Work out the finished part from the listing and answer in its coordinate system (mm). Face numbers are marked on the shaded views. Give positions to 0.01 mm unless a question says otherwise; leave off trailing zeros. Loops run counter-clockwise (first coordinate to the right, second up) from the corner with the lowest first, then second, coordinate; pieces in that order, holes last.
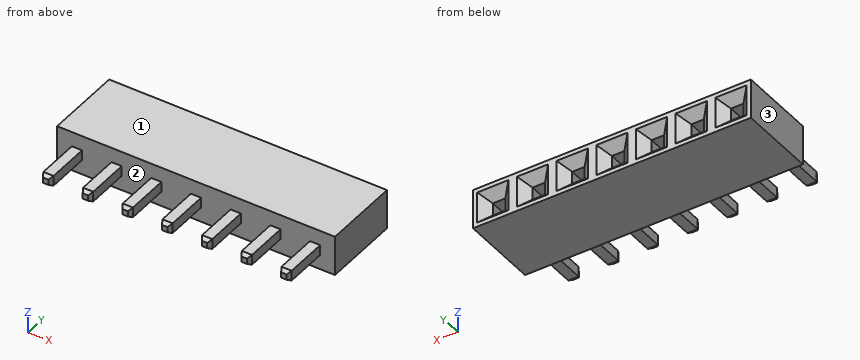
from build123d import *

# Parameters (mm, degrees)
SKETCH1_W                   = 2.54
SKETCH1_H                   = 2.54
BOSS_EXTRUDE1_DEPTH         = 5
SKETCH2_W                   = 0.65
SKETCH2_H                   = 0.65
BOSS_EXTRUDE2_DEPTH         = 3
CHAMFER1_SIZE               = 0.15
CHAMFER1_SIZE2              = 0.259807621
SKETCH3_W                   = 0.8
SKETCH3_H                   = 0.8
CUT_EXTRUDE1_DEPTH          = 3
CHAMFER2_SIZE               = 0.6
LPATTERN1_COUNT             = 7
LPATTERN1_PITCH             = 2.54
CHAMFER1_OF_LPATTERN1_SIZE2 = 0.15
CHAMFER1_OF_LPATTERN1_SIZE  = 0.259807621
CHAMFER2_OF_LPATTERN1_SIZE  = 0.6


with BuildPart() as part:
    # Sketch1 → Boss-Extrude1 (new body)
    with BuildSketch(Plane(origin=(0, 0, 0), x_dir=(1, 0, 0), z_dir=(0, 1, 0))):
        Rectangle(SKETCH1_W, SKETCH1_H)
    boss_extrude1 = extrude(amount=BOSS_EXTRUDE1_DEPTH)

    # Sketch2 → Boss-Extrude2 (add)
    with BuildSketch(Plane.XZ):
        Rectangle(SKETCH2_W, SKETCH2_H)
    boss_extrude2 = extrude(amount=BOSS_EXTRUDE2_DEPTH)

    # Chamfer1
    chamfer1_edges = [part.edges().sort_by_distance(p)[0] for p in [
        (0.325, -3, 0),
        (0, -3, 0.325),
        (-0.325, -3, 0),
        (0, -3, -0.325),
    ]]
    chamfer1_side = [part.faces().sort_by_distance(p)[0] for p in [
        (0, -3, 0),
    ]]
    chamfer(chamfer1_edges, length=CHAMFER1_SIZE, length2=CHAMFER1_SIZE2, reference=chamfer1_side[0])

    # Sketch3 → Cut-Extrude1 (cut)
    with BuildSketch(Plane(origin=(0, 5, 0), x_dir=(1, 0, 0), z_dir=(0, 1, 0))):
        Rectangle(SKETCH3_W, SKETCH3_H)
    cut_extrude1 = extrude(amount=-CUT_EXTRUDE1_DEPTH, mode=Mode.SUBTRACT)

    # Chamfer2
    chamfer2_edges = [part.edges().sort_by_distance(p)[0] for p in [
        (0.4, 5, 0),
        (0, 5, -0.4),
        (-0.4, 5, 0),
        (0, 5, 0.4),
    ]]
    chamfer(chamfer2_edges, length=CHAMFER2_SIZE)

    # LPattern1: Boss-Extrude1, Boss-Extrude2, Cut-Extrude1 ×7
    with Locations(*[(i * LPATTERN1_PITCH, 0, 0) for i in range(1, LPATTERN1_COUNT)]):
        add(boss_extrude1)
        add(boss_extrude2)
        add(cut_extrude1, mode=Mode.SUBTRACT)

    # Chamfer1 of LPattern1
    chamfer1_of_lpattern1_edges = [part.edges().sort_by_distance(p)[0] for p in [
        (2.865, -3, 0),
        (2.54, -3, 0.325),
        (2.215, -3, 0),
        (2.54, -3, -0.325),
        (5.405, -3, 0),
        (5.08, -3, 0.325),
        (4.755, -3, 0),
        (5.08, -3, -0.325),
        (7.945, -3, 0),
        (7.62, -3, 0.325),
        (7.295, -3, 0),
        (7.62, -3, -0.325),
        (10.485, -3, 0),
        (10.16, -3, 0.325),
        (9.835, -3, 0),
        (10.16, -3, -0.325),
        (13.025, -3, 0),
        (12.7, -3, 0.325),
        (12.375, -3, 0),
        (12.7, -3, -0.325),
        (15.565, -3, 0),
        (15.24, -3, 0.325),
        (14.915, -3, 0),
        (15.24, -3, -0.325),
    ]]
    chamfer(chamfer1_of_lpattern1_edges, length=CHAMFER1_OF_LPATTERN1_SIZE, length2=CHAMFER1_OF_LPATTERN1_SIZE2)

    # Chamfer2 of LPattern1
    chamfer2_of_lpattern1_edges = [part.edges().sort_by_distance(p)[0] for p in [
        (2.94, 5, 0),
        (2.54, 5, -0.4),
        (2.14, 5, 0),
        (2.54, 5, 0.4),
        (5.48, 5, 0),
        (5.08, 5, -0.4),
        (4.68, 5, 0),
        (5.08, 5, 0.4),
        (8.02, 5, 0),
        (7.62, 5, -0.4),
        (7.22, 5, 0),
        (7.62, 5, 0.4),
        (10.56, 5, 0),
        (10.16, 5, -0.4),
        (9.76, 5, 0),
        (10.16, 5, 0.4),
        (13.1, 5, 0),
        (12.7, 5, -0.4),
        (12.3, 5, 0),
        (12.7, 5, 0.4),
        (15.64, 5, 0),
        (15.24, 5, -0.4),
        (14.84, 5, 0),
        (15.24, 5, 0.4),
    ]]
    chamfer(chamfer2_of_lpattern1_edges, length=CHAMFER2_OF_LPATTERN1_SIZE)


solid = part.part
Item 1: Find section B-B, the plane y = -1.5. Write down the section's boundary in (x, z) (3 decimals).
Item 2: Consider line 1 (Z direction, x = 13, y = 4); line 2 (Z direction, x = 12.75, y = 4.5); line 3 (Y direction, x = 1.5, z = 0.1). Determine where each line is inside the solid, lowest interval first.
Item 3: Find section C-C, the plane x = 11. Write down the section's boundary in (y, z).
Item 4: Find section D-D, the plane y = 3.25. Give the number of separate pieces and of enclosed holes in the cut face, plus the area to 3 significant figures.
Item 5: Flat-ended cylindrical pins translate along their axes: pin 1 Ø0.6 at (x, z) = (2.5, 0) entering from +Y; pin 2 Ø0.5 at (x, y) = (2.5, -1) entering from -Z (3 decimals); pin 3 Ø0.9 at (x, z) = (15, 0) entering from +Y. Find the tip coordinate at first contact, or state that the pin passes through.
Item 6: Determine the mould class of the marked faces 1, 2 and 3 for opening direction X: released by +X, released by -X, zero draft, split by the parting line, or undercut.
Ans:
1. outline: (-0.325, -0.325) - (0.325, -0.325) - (0.325, 0.325) - (-0.325, 0.325) - close; (2.215, -0.325) - (2.865, -0.325) - (2.865, 0.325) - (2.215, 0.325) - close; (4.755, -0.325) - (5.405, -0.325) - (5.405, 0.325) - (4.755, 0.325) - close; (7.295, -0.325) - (7.945, -0.325) - (7.945, 0.325) - (7.295, 0.325) - close; (9.835, -0.325) - (10.485, -0.325) - (10.485, 0.325) - (9.835, 0.325) - close; (12.375, -0.325) - (13.025, -0.325) - (13.025, 0.325) - (12.375, 0.325) - close; (14.915, -0.325) - (15.565, -0.325) - (15.565, 0.325) - (14.915, 0.325) - close
2. line 1: z = -1.27 to -0.4, 0.4 to 1.27
2. line 2: z = -1.27 to -0.5, 0.5 to 1.27
2. line 3: y = 0 to 5
3. outline: (0, -1.27) - (5, -1.27) - (5, -1) - (4.84, -0.84) - (4.84, 0.84) - (5, 1) - (5, 1.27) - (0, 1.27) - close
4. separate pieces: 1
4. enclosed holes: 7
4. area: 40.7 mm2
5. pin 1: stops at y = 2
5. pin 2: stops at z = -0.325
5. pin 3: stops at y = 4.69
6. face 1: zero draft
6. face 2: undercut
6. face 3: released by -X
